from build123d import *

# Parameters (mm, degrees)
BOSS_EXTRUDE1_DEPTH = 80
CUT_EXTRUDE1_REACH  = 100.234
CUT_EXTRUDE2_DEPTH  = 80
CUT_EXTRUDE3_REACH  = 98.047
SKETCH5_R           = 4
CUT_EXTRUDE4_REACH  = 100.234
SKETCH6_R           = 4


with BuildPart() as part:
    # Sketch1 → Boss-Extrude1 (new body)
    with BuildSketch(Plane(origin=(0, 0, 0), x_dir=(0, 0, -1), z_dir=(1, 0, 0))):
        with BuildLine():
            Line((-40, 20), (-40, 5))
            ThreePointArc((-40, 5), (-38.535533906, 1.464466094), (-35, 0))
            Line((-35, 0), (0, 0))
            ThreePointArc((0, 0), (3.535533906, 1.464466094), (5, 5))
            Line((5, 5), (5, 30))
            ThreePointArc((5, 30), (3.535533906, 33.535533906), (0, 35))
            Line((0, 35), (-30, 35))
            Line((-30, 35), (-30, 30))
            Line((-30, 30), (-5, 30))
            ThreePointArc((-5, 30), (-1.464466094, 28.535533906), (0, 25))
            Line((0, 25), (0, 10))
            ThreePointArc((0, 10), (-1.464466094, 6.464466094), (-5, 5))
            Line((-5, 5), (-30, 5))
            ThreePointArc((-30, 5), (-33.535533906, 6.464466094), (-35, 10))
            Line((-35, 10), (-35, 20))
            Line((-35, 20), (-40, 20))
        make_face()
    extrude(amount=BOSS_EXTRUDE1_DEPTH)

    # Sketch2 → Cut-Extrude1 (cut, up to next)
    with BuildSketch(Plane(origin=(0, 0, -5), x_dir=(-1, 0, 0), z_dir=(0, 0, -1)), mode=Mode.PRIVATE) as cut_extrude1_sk1:
        with BuildLine():
            Line((-62.5, 22), (-17.5, 22))
            ThreePointArc((-17.5, 22), (-15.732233047, 21.267766953), (-15, 19.5))
            Line((-15, 19.5), (-15, 12.5))
            ThreePointArc((-15, 12.5), (-15.732233047, 10.732233047), (-17.5, 10))
            Line((-17.5, 10), (-62.5, 10))
            ThreePointArc((-62.5, 10), (-64.267766953, 10.732233047), (-65, 12.5))
            Line((-65, 12.5), (-65, 19.5))
            ThreePointArc((-65, 19.5), (-64.267766953, 21.267766953), (-62.5, 22))
        make_face()
    cut_extrude1_tool1 = extrude(cut_extrude1_sk1.sketch, amount=-CUT_EXTRUDE1_REACH, mode=Mode.PRIVATE) & part.part
    add(cut_extrude1_tool1.solids().sort_by_distance((40, 16, -5))[0], mode=Mode.SUBTRACT)

    # Sketch4 → Cut-Extrude2 (cut)
    with BuildSketch(Plane(origin=(0, 35, 0), x_dir=(1, 0, 0), z_dir=(0, 1, 0))):
        with BuildLine():
            Line((20, -40), (20, -33))
            ThreePointArc((20, -33), (21.464466094, -29.464466094), (25, -28))
            Line((25, -28), (55, -28))
            ThreePointArc((55, -28), (58.535533906, -29.464466094), (60, -33))
            Line((60, -33), (60, -40))
            Line((60, -40), (20, -40))
        make_face()
    extrude(amount=-CUT_EXTRUDE2_DEPTH, mode=Mode.SUBTRACT)

    # Sketch5 → Cut-Extrude3 (cut, up to next)
    with BuildSketch(Plane(origin=(0, 35, 0), x_dir=(1, 0, 0), z_dir=(0, 1, 0)), mode=Mode.PRIVATE) as cut_extrude3_sk1:
        with Locations(Location((10, -18, 0), (0, 0, 270))):
            Circle(SKETCH5_R)
    cut_extrude3_tool1 = extrude(cut_extrude3_sk1.sketch, amount=-CUT_EXTRUDE3_REACH, mode=Mode.PRIVATE) & part.part
    # Sketch5 → Cut-Extrude3 (cut, up to next)
    with BuildSketch(Plane(origin=(0, 35, 0), x_dir=(1, 0, 0), z_dir=(0, 1, 0)), mode=Mode.PRIVATE) as cut_extrude3_sk2:
        with Locations(Location((70, -18, 0), (0, 0, 270))):
            Circle(SKETCH5_R)
    cut_extrude3_tool2 = extrude(cut_extrude3_sk2.sketch, amount=-CUT_EXTRUDE3_REACH, mode=Mode.PRIVATE) & part.part
    # Sketch5 → Cut-Extrude3 (cut, up to next)
    with BuildSketch(Plane(origin=(0, 35, 0), x_dir=(1, 0, 0), z_dir=(0, 1, 0)), mode=Mode.PRIVATE) as cut_extrude3_sk3:
        with BuildLine():
            Line((20, -30), (21, -30))
            ThreePointArc((21, -30), (22.763932023, -28.527864045), (25, -28))
            Line((25, -28), (55, -28))
            ThreePointArc((55, -28), (57.236067977, -28.527864045), (59, -30))
            Line((59, -30), (60, -30))
            Line((60, -30), (60, -15))
            ThreePointArc((60, -15), (58.535533906, -11.464466094), (55, -10))
            Line((55, -10), (25, -10))
            ThreePointArc((25, -10), (21.464466094, -11.464466094), (20, -15))
            Line((20, -15), (20, -30))
        make_face()
    cut_extrude3_tool3 = extrude(cut_extrude3_sk3.sketch, amount=-CUT_EXTRUDE3_REACH, mode=Mode.PRIVATE) & part.part
    add(cut_extrude3_tool1.solids().sort_by_distance((10, 35, 18))[0], mode=Mode.SUBTRACT)
    add(cut_extrude3_tool2.solids().sort_by_distance((70, 35, 18))[0], mode=Mode.SUBTRACT)
    add(cut_extrude3_tool3.solids().sort_by_distance((40, 35, 19.237715))[0], mode=Mode.SUBTRACT)

    # Sketch6 → Cut-Extrude4 (cut, up to next)
    with BuildSketch(Plane.XY.offset(40), mode=Mode.PRIVATE) as cut_extrude4_sk1:
        with Locations((10, 14)):
            Circle(SKETCH6_R)
    cut_extrude4_tool1 = extrude(cut_extrude4_sk1.sketch, amount=-CUT_EXTRUDE4_REACH, mode=Mode.PRIVATE) & part.part
    # Sketch6 → Cut-Extrude4 (cut, up to next)
    with BuildSketch(Plane.XY.offset(40), mode=Mode.PRIVATE) as cut_extrude4_sk2:
        with Locations((70, 14)):
            Circle(SKETCH6_R)
    cut_extrude4_tool2 = extrude(cut_extrude4_sk2.sketch, amount=-CUT_EXTRUDE4_REACH, mode=Mode.PRIVATE) & part.part
    add(cut_extrude4_tool1.solids().sort_by_distance((10, 14, 40))[0], mode=Mode.SUBTRACT)
    add(cut_extrude4_tool2.solids().sort_by_distance((70, 14, 40))[0], mode=Mode.SUBTRACT)


solid = part.part
The model under review builds one solid part; all positions refer to its coordinate system, in mm. A direction names the side the tool comes from. Round coordinates to 2 decimals unless told otherwise and drop trailing zeros. Write each loop counter-clockwise with the first axis right and the second up, starting at its lowest first coordinate (ties: lowest second). Pieces come first, ordered by that corner, then holes. Notation, with made-up numbers: (59.25, 80) - (97.25, 80) arc R19 cw to (97.25, 111) - close; hole circle Ø3 at (37, 41). An arc over 180 degrees is marked (long way). One line per item, written item: value. Start each with the question number.
1. Clearance check with flat-ended pins moving along their axes: P1, Ø1.5, axis at x = 68.5, y = 33.5, coming from the +Z side; P2, Ø2, axis at x = 51, y = 28, coming from the +Z side; P3, Ø1, axis at x = 34.5, y = 29, coming from the +Z side. State where each tip first meets the part, or that it passes through.
2. Consider section B-B on y = 14. Write out the cut boundary in (x, z).
3. To check wall thickness, follow L1, parallel to X at y = 32.6, z = 18; L2, parallel to Y at x = 69.5, z = 13; L3, parallel to Z at x = 50, y = 24.5. State the ranges of each line that lie inside material, in increasing order. Write a range as from..to.
4. Consider section C-C on z = 18. Write out the cut boundary in (x, y), and give its area (3 significant figures).
5. Consider section A-A on x = 37.5. Write out the cut boundary in (y, z), and give its area (3 significant figures).
6. Consider section D-D on y = 8. Write out the cut boundary in (x, z), and give its area (3 significant figures).
7. Machinability: for faces 1 (the face through (39, 30, 9)), 2 (the face through (70, 20, 37)), 3 (the face through (64.248, 10.713, -2.535)), 4 (the face through (20, 10, 37)), which of the approach directions +Z, -Z, +X, -X, +Y, -Y give a long, thin tool a straight path to every point of the face, cutting with its end or side? Answer none if there is none.
Checks:
1. P1: stops at z = 30
1. P2: stops at z = 2
1. P3: stops at z = 2.82
2. outline: (0, -5) - (15, -5) - (15, 0) - (0, 0) - close; (0, 35) - (6, 35) - (6, 40) - (0, 40) - close; (14, 35) - (20, 35) - (20, 40) - (14, 40) - close; (60, 35) - (66, 35) - (66, 40) - (60, 40) - close; (65, -5) - (80, -5) - (80, 0) - (65, 0) - close; (74, 35) - (80, 35) - (80, 40) - (74, 40) - close
3. L1: x = 0..6, 14..20, 60..66, 74..80
3. L2: y = 0..5, 30..35
3. L3: z = -5..0
4. outline: (0, 0) - (80, 0) - (80, 5) - (0, 5) - close; (0, 30) - (6, 30) - (6, 35) - (0, 35) - close; (14, 30) - (20, 30) - (20, 35) - (14, 35) - close; (60, 30) - (66, 30) - (66, 35) - (60, 35) - close; (74, 30) - (80, 30) - (80, 35) - (74, 35) - close
4. area: 520 mm^2
5. outline: (0, 0) arc R5 ccw to (5, -5) - (10, -5) - (10, 0) arc R5 cw to (5, 5) - (5, 28) - (0, 28) - close; (22, -5) - (30, -5) arc R5 ccw to (35, 0) - (35, 10) - (30, 10) - (30, 5) arc R5 cw to (25, 0) - (22, 0) - close
5. area: 305 mm^2
6. outline: (0, -5) - (80, -5) - (80, 0.42) - (0, 0.42) - close; (0, 34.58) - (20, 34.58) - (20, 40) - (0, 40) - close; (60, 34.58) - (80, 34.58) - (80, 40) - (60, 40) - close
6. area: 650 mm^2
7. face 1: +Z, +X, -X
7. face 2: +Z, +X, -X, +Y
7. face 3: -Z
7. face 4: +Z, +Y, -Y
